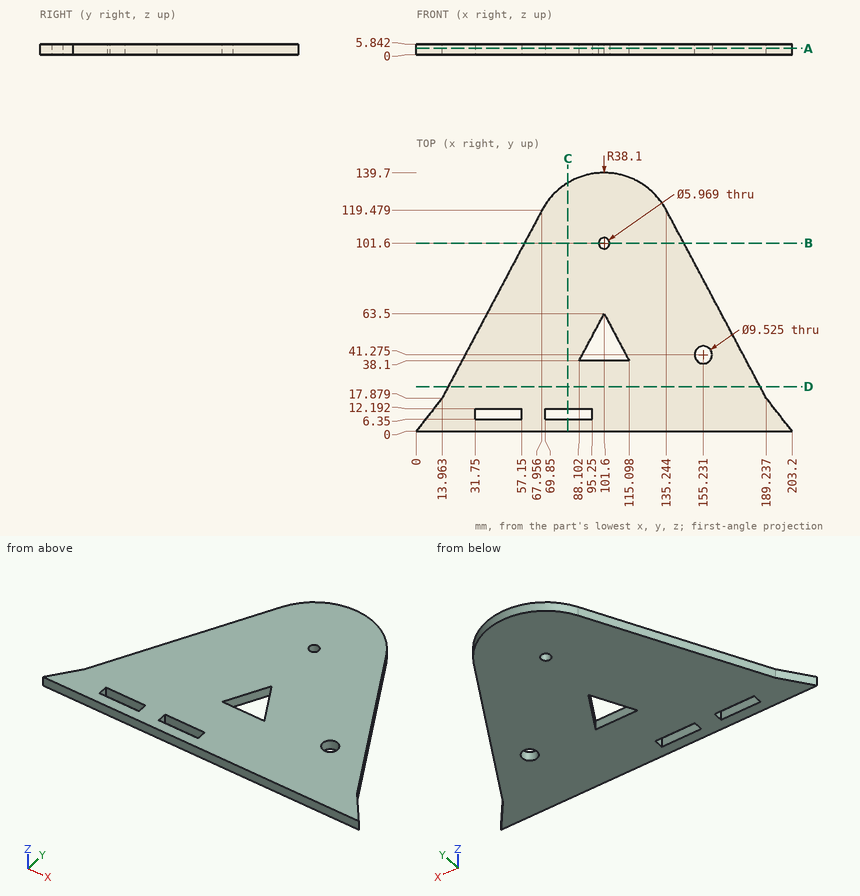
Answer from the drawing. Dimensions are ordinates in mm from the lowest x, y and z of the part. Round coordinates to 2 decimals unless told otherwise and drop trailing zeros. Write each loop counter-clockwise with the first axis right and the second up, starting at its lowest first coordinate (ties: lowest second). Pieces come first, ordered by that corner, then holes. Notation, with made-up numbers: (-5.75, -8) -> (18.25, -8) arc R18 ccw to (18.25, 6) -> close; hole circle Ø3 at (61, 10.25). An arc over 180 degrees is marked (long way). Write each question's results on one line, items separated by ' | '.
1) The part is cut by section D-D (y = 24). Write down the section's boundary in (x, z) (1 decimal), and give its area (3 significant figures).
Findings:
outline: (17.2, 0) -> (186, 0) -> (186, 5.8) -> (17.2, 5.8) -> close | area: 986 mm²
2) The part is cut by section B-B (y = 101.6). Write down the section's boundary in (x, z) (1 decimal).
Findings:
outline: (58.5, 0) -> (98.6, 0) -> (98.6, 5.8) -> (58.5, 5.8) -> close; (104.6, 0) -> (144.7, 0) -> (144.7, 5.8) -> (104.6, 5.8) -> close
3) Flat-ended cylindrical pins translate along their axes: pin 1 (2 mm diameter, centred on y = 56, z = 3.5, fed in from +X); pin 2 (1.8 mm diameter, centred on x = 98, z = 4, fed in from +Y); pin 3 (1 mm diameter, centred on x = 93.5, z = 0.5, fed in from +Y) (1 decimal). Find the tip coordinate at first contact, or state that the pin passes through.
Findings:
pin 1: stops at x = 169.51 | pin 2: stops at y = 139.6 | pin 3: stops at y = 138.9
4) The part is cut by section A-A (z = 3.45). State how many separate pieces and enclosed holes the cut face has, and give its area (3 significant figures).
Findings:
separate pieces: 1 | enclosed holes: 5 | area: 15,900 mm²
5) Consider line 1 along Y through (x, z) = (101.6, 3.65) (1 decimal); line 2 along X through (y, z) = (43, 0.8) (1 decimal); line 3 along Y through (x, z) = (101.5, 2.25) (1 decimal). Determine where each line is inside the solid, lowest interval first. Write a range as [from, to].
Findings:
line 1: y = [0, 38.1], [63.5, 98.6], [104.6, 139.7] | line 2: x = [27.3, 90.7], [112.5, 150.8], [159.7, 175.9] | line 3: y = [0, 38.1], [63.3, 98.6], [104.6, 139.7]
6) The part is cut by section C-C (x = 82). Write down the section's boundary in (y, z).
Findings:
outline: (0, 0) -> (6.35, 0) -> (6.35, 5.84) -> (0, 5.84) -> close; (12.19, 0) -> (134.27, 0) -> (134.27, 5.84) -> (12.19, 5.84) -> close
